For this review, take the finished solid that the model builds, in its own axes (mm). A direction names the side the tool comes from. Coordinates: 2 decimals unless noted, no trailing zeros. Order: outer loops, then holes, each group sorted by start corner. A loop starts at its lowest first (then second) coordinate and runs counter-clockwise, first axis right, second up. Notation, with made-up numbers: (0.5, 63.25) - (41.5, 63.25) arc R31 ccw to (41.5, 87.25) - close; hole circle Ø4 at (76.25, 48.25). An arc over 180 degrees is marked (long way). One line per item, written item: value. Start each with the question number.
(1) To check wall thickness, follow line 1 along X through (y, z) = (0.35, 1.5); line 2 along Y through (x, z) = (-8, -21); line 3 along Z through (x, y) = (0, -2.05). State the ranges of each line that lie inside material, in increasing order.
(2) Consider section D-D on x = 20. Write out the cut boundary in (y, z).
(3) Clearance check with flat-ended pins moving along their axes: pin 1 (13 mm diameter, centred on x = 17, z = 0, fed in from +Y); pin 2 (3.5 mm diameter, centred on x = -22.5, z = 2, fed in from +Y). State where each tip first meets the part, or that it passes through.
(4) Consider section B-B on z = 3.5. Write out the cut boundary in (x, y), then the cut area to 3 significant figures.
(5) Consider section A-A on y = 1.9. Write out the cut boundary in (x, z), then the cut area to 3 significant figures.
(6) Consider section C-C on y = -0.8. Write out the cut boundary in (x, z), then the cut area to 3 significant figures.
(7) Mouldability with a two-part tool opening along Z and no side actions: class faces 1 (the cylindrical face through (-20, -1.5, -5.1)), 2 (the flat face through (14.61, 1.52, -10.11)), 3 (the flat face through (0, -1, 7.5)) as released by +Z, released by -Z, zero draft, split by the parting line, or undercut.
(8) For faces 4 (the flat face through (-23, 0, -1)), 5 (the flat face through (-21.6, -1, 0)), 6 (the cylindrical face through (-29.14, -1.52, -21.6)), 7 (the flat face through (0, -1, -22.5)), 8 (the flat face through (0, 0, -17)), list the 3-axis set-ups (+Z, -Z, +X, -X, +Y, -Y) from which the entire face can be reached by the end or side of a thin tool; tool diameter is ignored.
```python
from build123d import *

# Parameters (mm, degrees)
BOSS_EXTRUDE1_DEPTH = 3
SKETCH4_W           = 60
SKETCH4_H           = 30
BOSS_EXTRUDE2_DEPTH = 3
FILLET1_R           = 3
CUT_EXTRUDE1_DEPTH  = 38.976966704
BOSS_EXTRUDE3_DEPTH = 3
CUT_EXTRUDE2_DEPTH  = 3
FILLET2_R           = 1


with BuildPart() as part:
    # Sketch2 → Boss-Extrude1 (new body)
    with BuildSketch(Plane(origin=(0, 0, 0), x_dir=(1, 0, 0), z_dir=(0, 1, 0))):
        with BuildLine():
            Line((-30, -7.5), (30, -7.5))
            Line((30, -7.5), (30, 11.664728706))
            ThreePointArc((30, 11.664728706), (29.572172135, 12.484862261), (28.654761905, 12.60324384))
            ThreePointArc((28.654761905, 12.60324384), (0, 7.5), (-28.654761905, 12.60324384))
            ThreePointArc((-28.654761905, 12.60324384), (-29.572172135, 12.484862261), (-30, 11.664728706))
            Line((-30, 11.664728706), (-30, -7.5))
        make_face()
    extrude(amount=BOSS_EXTRUDE1_DEPTH)

    # Sketch4 → Boss-Extrude2 (add)
    with BuildSketch(Plane.XZ):
        with Locations((0, -7.5)):
            Rectangle(SKETCH4_W, SKETCH4_H)
    extrude(amount=BOSS_EXTRUDE2_DEPTH)

    # Fillet1
    fillet1_edges = [part.edges().sort_by_distance(p)[0] for p in [
        (30, -1.5, -22.5),
        (30, 0, 7.5),
        (-30, 0, 7.5),
        (-30, -1.5, -22.5),
    ]]
    fillet(fillet1_edges, radius=FILLET1_R)

    # Sketch5 → Cut-Extrude1 (cut, through all)
    with BuildSketch(Plane(origin=(0, 3, 0), x_dir=(1, 0, 0), z_dir=(0, 1, 0))):
        with BuildLine():
            Line((1.6, 3.5), (1.6, -4.5))
            ThreePointArc((1.6, -4.5), (0, -6.1), (-1.6, -4.5))
            Line((-1.6, -4.5), (-1.6, 3.5))
            ThreePointArc((-1.6, 3.5), (0, 5.1), (1.6, 3.5))
        make_face()
        with BuildLine():
            Line((21.6, 3.5), (21.6, -4.5))
            ThreePointArc((21.6, -4.5), (20, -6.1), (18.4, -4.5))
            Line((18.4, -4.5), (18.4, 3.5))
            ThreePointArc((18.4, 3.5), (20, 5.1), (21.6, 3.5))
        make_face()
        with BuildLine():
            Line((-21.6, 3.5), (-21.6, -4.5))
            ThreePointArc((-21.6, -4.5), (-20, -6.1), (-18.4, -4.5))
            Line((-18.4, -4.5), (-18.4, 3.5))
            ThreePointArc((-18.4, 3.5), (-20, 5.1), (-21.6, 3.5))
        make_face()
    extrude(amount=-CUT_EXTRUDE1_DEPTH, mode=Mode.SUBTRACT)

    # Sketch6 → Boss-Extrude3 (add)
    with BuildSketch(Plane(origin=(0, 3, 0), x_dir=(1, 0, 0), z_dir=(0, 1, 0))):
        with BuildLine():
            Line((0, 7.5), (-28.824143961, 12.649144601))
            ThreePointArc((-28.824143961, 12.649144601), (-29.64192833, 12.43149335), (-30, 11.664728706))
            Line((-30, 11.664728706), (-30, -4.5))
            ThreePointArc((-30, -4.5), (-29.121320344, -6.621320344), (-27, -7.5))
            Line((-27, -7.5), (27, -7.5))
            ThreePointArc((27, -7.5), (29.121320344, -6.621320344), (30, -4.5))
            Line((30, -4.5), (30, 11.664728706))
            ThreePointArc((30, 11.664728706), (29.64192833, 12.43149335), (28.824143961, 12.649144601))
            Line((28.824143961, 12.649144601), (0, 7.5))
        make_face()
        with BuildLine():
            Line((-18.4, -4.5), (-18.4, 3.5))
            ThreePointArc((-18.4, 3.5), (-20, 5.1), (-21.6, 3.5))
            Line((-21.6, 3.5), (-21.6, -4.5))
            ThreePointArc((-21.6, -4.5), (-20, -6.1), (-18.4, -4.5))
        make_face(mode=Mode.SUBTRACT)
        with BuildLine():
            Line((1.6, -4.5), (1.6, 3.5))
            ThreePointArc((1.6, 3.5), (0, 5.1), (-1.6, 3.5))
            Line((-1.6, 3.5), (-1.6, -4.5))
            ThreePointArc((-1.6, -4.5), (0, -6.1), (1.6, -4.5))
        make_face(mode=Mode.SUBTRACT)
        with BuildLine():
            Line((21.6, -4.5), (21.6, 3.5))
            ThreePointArc((21.6, 3.5), (20, 5.1), (18.4, 3.5))
            Line((18.4, 3.5), (18.4, -4.5))
            ThreePointArc((18.4, -4.5), (20, -6.1), (21.6, -4.5))
        make_face(mode=Mode.SUBTRACT)
    extrude(amount=-BOSS_EXTRUDE3_DEPTH)

    # Sketch7 → Cut-Extrude2 (cut)
    with BuildSketch(Plane(origin=(0, 3, 0), x_dir=(1, 0, 0), z_dir=(0, 1, 0))):
        with BuildLine():
            Line((-15, 3.5), (-15, -15.7))
            ThreePointArc((-15, -15.7), (-20, -20.7), (-25, -15.7))
            Line((-25, -15.7), (-25, 3.5))
            ThreePointArc((-25, 3.5), (-20, 8.5), (-15, 3.5))
        make_face()
        with BuildLine():
            Line((25, 3.5), (25, -15.7))
            ThreePointArc((25, -15.7), (20, -20.7), (15, -15.7))
            Line((15, -15.7), (15, 3.5))
            ThreePointArc((15, 3.5), (20, 8.5), (25, 3.5))
        make_face()
    extrude(amount=-CUT_EXTRUDE2_DEPTH, mode=Mode.SUBTRACT)

    # Fillet2
    fillet2_edges = [part.edges().sort_by_distance(p)[0] for p in [
        (-15, 1.5, 7.5),
        (-25, 1.5, 7.5),
        (25, 1.5, 7.5),
        (15, 1.5, 7.5),
    ]]
    fillet(fillet2_edges, radius=FILLET2_R)


solid = part.part
```
Geometry check:
1. line 1: x = -30 to -25, -15 to -1.6, 1.6 to 15, 25 to 30
1. line 2: y = -3 to 0
1. line 3: z = -22.5 to -5.1, 6.1 to 7.5
2. outline: (-3, -22.5) - (0, -22.5) - (0, -11.07) - (3, -11.07) - (3, -8.5) - (0, -8.5) - (0, -5.1) - (-3, -5.1) - close; (-3, 6.1) - (0, 6.1) - (0, 7.5) - (-3, 7.5) - close
3. pin 1: stops at y = 3
3. pin 2: stops at y = 0
4. outline: (-30, -3) - (-21.6, -3) - (-21.6, 0) - (-25, 0) - (-25, 3) - (-30, 3) - close; (-18.4, -3) - (-1.6, -3) - (-1.6, 3) - (-15, 3) - (-15, 0) - (-18.4, 0) - close; (1.6, -3) - (18.4, -3) - (18.4, 0) - (15, 0) - (15, 3) - (1.6, 3) - close; (21.6, -3) - (30, -3) - (30, 3) - (25, 3) - (25, 0) - (21.6, 0) - close
4. area: 262 mm^2
5. outline: (-30, -11.66) arc R1 ccw to (-28.82, -12.65) - (0, -7.5) - (28.82, -12.65) arc R1 ccw to (30, -11.66) - (30, 4.5) arc R3 ccw to (27, 7.5) - (26, 7.5) arc R1 ccw to (25, 6.5) - (25, -3.5) arc R5 cw to (15, -3.5) - (15, 6.5) arc R1 ccw to (14, 7.5) - (-14, 7.5) arc R1 ccw to (-15, 6.5) - (-15, -3.5) arc R5 cw to (-25, -3.5) - (-25, 6.5) arc R1 ccw to (-26, 7.5) - (-27, 7.5) arc R3 ccw to (-30, 4.5) - close; hole (-1.6, -3.5) arc R1.6 ccw to (1.6, -3.5) - (1.6, 4.5) arc R1.6 ccw to (-1.6, 4.5) - close
5. area: 723 mm^2
6. outline: (-30, -19.5) arc R3 ccw to (-27, -22.5) - (27, -22.5) arc R3 ccw to (30, -19.5) - (30, 4.5) arc R3 ccw to (27, 7.5) - (-27, 7.5) arc R3 ccw to (-30, 4.5) - close; hole (-21.6, -3.5) arc R1.6 ccw to (-18.4, -3.5) - (-18.4, 4.5) arc R1.6 ccw to (-21.6, 4.5) - close; hole (-1.6, -3.5) arc R1.6 ccw to (1.6, -3.5) - (1.6, 4.5) arc R1.6 ccw to (-1.6, 4.5) - close; hole (18.4, -3.5) arc R1.6 ccw to (21.6, -3.5) - (21.6, 4.5) arc R1.6 ccw to (18.4, 4.5) - close
6. area: 1,690 mm^2
7. face 1: undercut
7. face 2: released by -Z
7. face 3: released by +Z
8. face 4: +Z, +Y
8. face 5: +Y, -Y
8. face 6: -Z, -X, +Y, -Y
8. face 7: -Z, +X, -X, +Y, -Y
8. face 8: -Z, +Y
